```python
from build123d import *

# Parameters (mm, degrees)
F0_W     = 25.4
F0_H     = 25.4
F1_DEPTH = 25.4
F2_R     = 11.43
F3_DEPTH = 25.401
F4_R     = 11.43
F5_DEPTH = 25.401
F6_R     = 11.43
F7_DEPTH = 25.401


with BuildPart() as f1:
    # F0 (on Top) → F1 (new body)
    with BuildSketch(Plane.XY):
        with Locations((12.7, 12.7)):
            Rectangle(F0_W, F0_H)
    extrude(amount=F1_DEPTH)

    # F2 (on face) → F3 (cut, through all)
    with BuildSketch(Plane.XY.offset(25.4)):
        with Locations((12.7, 12.7)):
            Circle(F2_R)
    extrude(amount=-F3_DEPTH, mode=Mode.SUBTRACT)

    # F4 (on face) → F5 (cut, through all)
    with BuildSketch(Plane(origin=(0, 0, 0), x_dir=(0, -1, 0), z_dir=(-1, 0, 0))):
        with Locations((-12.7, 12.7)):
            Circle(F4_R)
    extrude(amount=-F5_DEPTH, mode=Mode.SUBTRACT)

    # F6 (on face) → F7 (cut, through all)
    with BuildSketch(Plane(origin=(0, 25.4, 0), x_dir=(-1, 0, 0), z_dir=(0, 1, 0))):
        with Locations((-12.7, 12.7)):
            Circle(F6_R)
    extrude(amount=-F7_DEPTH, mode=Mode.SUBTRACT)


solid = f1.part
```
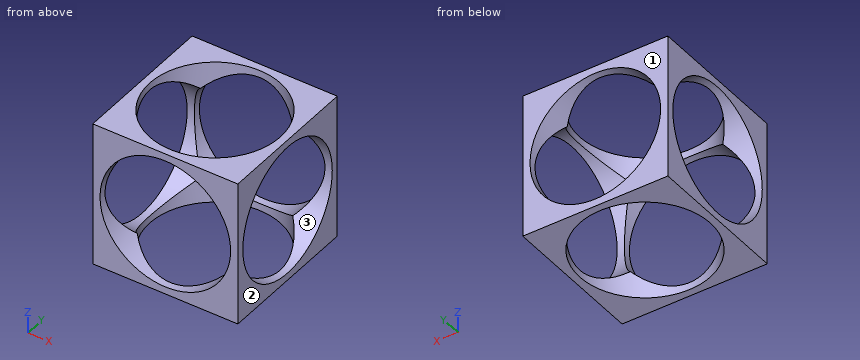
Check sheet for the modelled part. Datum: model origin and axes. Units: mm. Face numbers are marked on the shaded views. Give positions to 0.01 mm unless a question says otherwise; leave off trailing zeros. Write each loop counter-clockwise with the first axis right and the second up, starting at its lowest first coordinate (ties: lowest second). Pieces come first, ordered by that corner, then holes.
Item 1: Cross-section at A-A (y = 12.7). Enter the section's corners in (x, z), and give its area (3 significant figures).
Item 2: Cross-section at C-C (z = 4). Enter the section's corners in (x, y), and give its area (3 significant figures).
Item 3: Draft check along Y on the marked faces 1, 2 and 3. Enter one of: released by +Y, released by -Y, zero draft, split by the parting line, or undercut.
Item 4: Scan lines: L1, parallel to Y at x = 12.7, z = 1.05; L2, parallel to Z at x = 24, y = 6.5. Record each from-to range of solid material in increasing order.
Item 5: Cross-section at D-D (x = 22.75). Enter the section's corners in (y, z).
Report:
1. outline: (0, 0) - (1.27, 0) - (1.27, 1.27) - (0, 1.27) - close; (0, 24.13) - (1.27, 24.13) - (1.27, 25.4) - (0, 25.4) - close; (24.13, 0) - (25.4, 0) - (25.4, 1.27) - (24.13, 1.27) - close; (24.13, 24.13) - (25.4, 24.13) - (25.4, 25.4) - (24.13, 25.4) - close
1. area: 6.45 mm2
2. outline: (0, 0) - (5.29, 0) - (5.29, 4) arc R11.43 cw to (4, 5.29) - (0, 5.29) - close; (0, 20.11) - (4, 20.11) arc R11.43 cw to (5.29, 21.4) - (5.29, 25.4) - (0, 25.4) - close; (20.11, 0) - (25.4, 0) - (25.4, 5.29) - (21.4, 5.29) arc R11.43 cw to (20.11, 4) - close; (20.11, 21.4) arc R11.43 cw to (21.4, 20.11) - (25.4, 20.11) - (25.4, 25.4) - (20.11, 25.4) - close
2. area: 108 mm2
3. face 1: released by +Y
3. face 2: zero draft
3. face 3: undercut
4. L1: y = 0 to 1.27, 24.13 to 25.4
4. L2: z = 0 to 3.1, 22.3 to 25.4
5. outline: (0, 0) - (7.26, 0) - (7.26, 2.65) arc R11.43 cw to (2.65, 7.26) - (0, 7.26) - close; (0, 18.14) - (2.65, 18.14) arc R11.43 cw to (7.26, 22.75) - (7.26, 25.4) - (0, 25.4) - close; (18.14, 0) - (25.4, 0) - (25.4, 7.26) - (22.75, 7.26) arc R11.43 cw to (18.14, 2.65) - close; (18.14, 22.75) arc R11.43 cw to (22.75, 18.14) - (25.4, 18.14) - (25.4, 25.4) - (18.14, 25.4) - close
